Part print with two shaded views. Sizes in mm from the minimum x, y, z corner. Round coordinates to 2 decimals unless told otherwise and drop trailing zeros. Order: outer loops, then holes, each group sorted by start corner. A loop starts at its lowest first (then second) coordinate and runs counter-clockwise, first axis right, second up. Notation, with made-up numbers: M 76.5,50 L 124.5,50 A36 ccw 124.5,88 Z; hole C -25,3.25 d10. An arc over 180 degrees is marked long. Return JSON: item names as keys, results as strings. Group by question number.
Item 1: Probe line 1 along X through (y, z) = (3, 12.75); line 2 along X through (y, z) = (3.55, 16.75); line 3 along Z through (x, y) = (60, 0.6). List the from-to ranges inside material, lowest first.
Item 2: Pin check, flat tip, straight feed: pin 1 Ø5 at (x, z) = (41.5, 7.5) entering from -Y. Stop position of the tip, or through.
Item 3: Slice it at A-A on y = 1.6. Write the cut outline in (x, z).
Item 4: Slice it at C-C on x = 47. Write the cut outline in (y, z).
Item 5: Slice it at B-B on z = 17.5. Write the cut outline in (x, y) (1 decimal).
Item 6: Slice it at D-D on x = 78. Write the cut outline in (y, z).
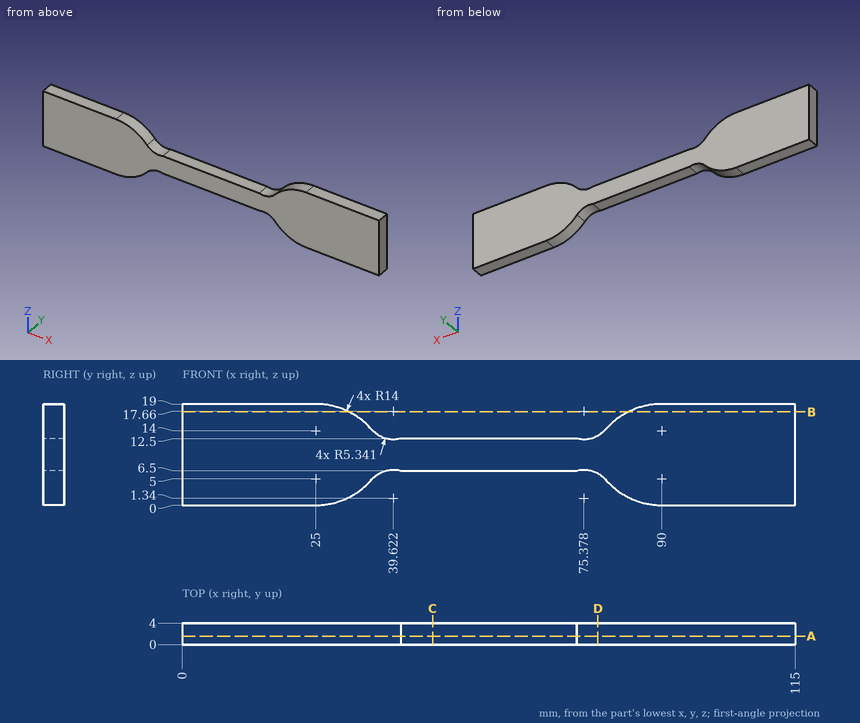
Output values:
{
 "1": {"line 1": "0 to 37.52, 77.48 to 115", "line 2": "0 to 32.61, 82.39 to 115", "line 3": "6.5 to 12.5"},
 "2": {"pin 1": "y = 0"},
 "3": {"outline": "M 0,0 L 25,0 A14 ccw 35.58,4.84 A5.34 cw 41,6.5 L 74,6.5 A5.34 cw 79.42,4.84 A14 ccw 90,0 L 115,0 L 115,19 L 90,19 A14 ccw 79.42,14.16 A5.34 cw 74,12.5 L 41,12.5 A5.34 cw 35.58,14.16 A14 ccw 25,19 L 0,19 Z"},
 "4": {"outline": "M 0,6.5 L 4,6.5 L 4,12.5 L 0,12.5 Z"},
 "5": {"outline": "M 0,0 L 31.3,0 L 31.3,4 L 0,4 Z; M 83.7,0 L 115,0 L 115,4 L 83.7,4 Z"},
 "6": {"outline": "M 0,5.99 L 4,5.99 L 4,13.01 L 0,13.01 Z"}
}
